from build123d import *

# Parameters (mm, degrees)
F0_W          = 25.4
F0_H          = 25.4
F1_DEPTH      = 12.7
F1_DEPTH_BACK = 12.7
F2_R          = 4.445
F8_DEPTH      = 25.4
F4_R          = 4.445
F9_DEPTH      = 25.4
F6_R          = 4.445
F10_DEPTH     = 25.4
F2_R_2        = 6.35
F11_DEPTH     = 3.175
F3_R          = 6.35
F3_R_2        = 4.445
F12_DEPTH     = 3.175
F4_R_2        = 6.35
F13_DEPTH     = 3.175
F5_R          = 6.35
F5_R_2        = 4.445
F14_DEPTH     = 3.175
F6_R_2        = 6.35
F15_DEPTH     = 3.175
F7_R          = 6.35
F7_R_2        = 4.445
F16_DEPTH     = 3.175
F17_SIZE      = 2.54


with BuildPart() as f1:
    # F0 (on Front) → F1 (new body, two sides)
    with BuildSketch(Plane.XZ) as f1_sk:
        Rectangle(F0_W, F0_H)
    extrude(amount=F1_DEPTH)
    extrude(f1_sk.sketch, amount=-F1_DEPTH_BACK)

    # F2 (on face) → F8 (cut)
    with BuildSketch(Plane.XY.offset(12.7)):
        Circle(F2_R)
    extrude(amount=-F8_DEPTH, mode=Mode.SUBTRACT)

    # F4 (on face) → F9 (cut)
    with BuildSketch(Plane.XZ.offset(12.7)):
        Circle(F4_R)
    extrude(amount=-F9_DEPTH, mode=Mode.SUBTRACT)

    # F6 (on face) → F10 (cut)
    with BuildSketch(Plane.YZ.offset(12.7)):
        Circle(F6_R)
    extrude(amount=-F10_DEPTH, mode=Mode.SUBTRACT)

    # F2 (on face) → F11 (cut)
    with BuildSketch(Plane.XY.offset(12.7)):
        Circle(F2_R_2)
        Circle(F2_R, mode=Mode.SUBTRACT)
    extrude(amount=-F11_DEPTH, mode=Mode.SUBTRACT)

    # F3 (on face) → F12 (cut)
    with BuildSketch(Plane(origin=(0, 0, -12.7), x_dir=(1, 0, 0), z_dir=(0, 0, -1))):
        Circle(F3_R)
        Circle(F3_R_2, mode=Mode.SUBTRACT)
    extrude(amount=-F12_DEPTH, mode=Mode.SUBTRACT)

    # F4 (on face) → F13 (cut)
    with BuildSketch(Plane.XZ.offset(12.7)):
        Circle(F4_R_2)
        Circle(F4_R, mode=Mode.SUBTRACT)
    extrude(amount=-F13_DEPTH, mode=Mode.SUBTRACT)

    # F5 (on face) → F14 (cut)
    with BuildSketch(Plane(origin=(0, 12.7, 0), x_dir=(-1, 0, 0), z_dir=(0, 1, 0))):
        Circle(F5_R)
        Circle(F5_R_2, mode=Mode.SUBTRACT)
    extrude(amount=-F14_DEPTH, mode=Mode.SUBTRACT)

    # F6 (on face) → F15 (cut)
    with BuildSketch(Plane.YZ.offset(12.7)):
        Circle(F6_R_2)
        Circle(F6_R, mode=Mode.SUBTRACT)
    extrude(amount=-F15_DEPTH, mode=Mode.SUBTRACT)

    # F7 (on face) → F16 (cut)
    with BuildSketch(Plane(origin=(-12.7, 0, 0), x_dir=(0, -1, 0), z_dir=(-1, 0, 0))):
        Circle(F7_R)
        Circle(F7_R_2, mode=Mode.SUBTRACT)
    extrude(amount=-F16_DEPTH, mode=Mode.SUBTRACT)

    # F17
    f17_edges = [f1.edges().sort_by_distance(p)[0] for p in [
        (12.7, -12.7, 0),
        (0, -12.7, -12.7),
        (-12.7, -12.7, 0),
        (0, -12.7, 12.7),
        (12.7, 0, -12.7),
        (-12.7, 0, -12.7),
        (0, 12.7, -12.7),
        (12.7, 12.7, 0),
        (12.7, 0, 12.7),
        (0, 12.7, 12.7),
        (-12.7, 0, 12.7),
        (-12.7, 12.7, 0),
    ]]
    chamfer(f17_edges, length=F17_SIZE)


solid = f1.part
Design review of the part built by this model. Coordinates are the model's own, in mm. A direction names the side the tool comes from. Give positions to 0.01 mm unless a question says otherwise; leave off trailing zeros. Order: outer loops, then holes, each group sorted by start corner. A loop starts at its lowest first (then second) coordinate and runs counter-clockwise, first axis right, second up. Notation, with made-up numbers: (66, -30) - (77, -30) arc R17 ccw to (77, -25) - close; hole circle Ø4 at (-36, -0.75). An arc over 180 degrees is marked (long way). Use CSV: the item, a comma, the result in double quotes. Start each with the question number.
Q1. Take a section at C-C (y = 0). Count the separate pieces of the cut face and the enclosed holes in it, and give its area (3 significant figures).
Q2. For P1, Ø6.5, axis at x = -2.5, y = -1.5, coming from the -Z side (3 decimals); P2, Ø10, axis at x = 0, y = 0, coming from the +Z side (3 decimals); P3, Ø11.5, axis at x = 0, z = 0, coming from the +Y side (3 decimals), all flat-tipped, find the tip position at first contact; note any pin that passes through.
Q3. Draft analysis for pull direction Y (two halves, no side actions). For faces 1 (the face through (11.41, -0.14, 11.45)), 2 (the face through (-1.38, -6.2, 11.13)), 3 (the face through (-11.13, 10.93, 10.96)), state which applies: pulls with the +Y half, pulls with the -Y half, needs draft (parallel to the pull), parting line crosses it, or undercut.
Q4. For line 1 (Z direction, x = -7.25, y = 0) (3 decimals), list the stretches that pass through material, from the lowest coordinate up.
Q5. Take a section at A-A (x = -7.5). State the section outline as (y, z) points (3 decimals).
Q6. Machinability: for faces 4 (the face through (7.09, -4.44, 0.2)), 5 (the face through (-11.13, 1.38, -6.2)), 6 (the face through (-1.38, -11.13, -6.2)), 7 (the face through (1.38, 11.13, -6.2)), 8 (the face through (-4.44, -7.09, 0.2)), which of the approach directions +Z, -Z, +X, -X, +Y, -Y give a long, thin tool a straight path to every point of the face, cutting with its end or side? Answer none if there is none.
Calculated:
1,separate pieces,"4"
1,enclosed holes,"0"
1,area,"211 mm²"
2,P1,"stops at z = -9.525"
2,P2,"stops at z = 9.525"
2,P3,"stops at y = 9.525"
3,face 1,"needs draft"
3,face 2,"undercut"
3,face 3,"pulls with the +Y half"
4,line 1,"z = -12.7 to -4.445, 4.445 to 12.7"
5,outline,"(-12.7, -10.16) - (-10.16, -12.7) - (10.16, -12.7) - (12.7, -10.16) - (12.7, 10.16) - (10.16, 12.7) - (-10.16, 12.7) - (-12.7, 10.16) - close; hole circle Ø8.89 at (0, 0)"
6,face 4,"+X, -X"
6,face 5,"-X"
6,face 6,"-Y"
6,face 7,"+Y"
6,face 8,"+Y, -Y"
